from build123d import *
from build123d.topology import SkipClean

# Parameters (mm, degrees)
BOSS_EXTRUDE1_DEPTH  = 2
BOSS_EXTRUDE2_START  = 4.75
BOSS_EXTRUDE2_DEPTH  = 4.75
BOSS_EXTRUDE3_START  = 2
SKETCH3_R            = 1.7
BOSS_EXTRUDE3_DEPTH  = 2
SKETCH4_R            = 2.2
SKETCH4_R_2          = 1.7
BOSS_EXTRUDE4_DEPTH  = 0.5
CHAMFER1_SIZE        = 0.5
SKETCH5_W            = 7.5
SKETCH5_H            = 3
BOSS_EXTRUDE5_DEPTH  = 2
BOSS_EXTRUDE6_DEPTH  = 6.75
BOSS_EXTRUDE8_DEPTH  = 6.75
SKETCH10_W           = 15
SKETCH10_H           = 3
BOSS_EXTRUDE9_DEPTH  = 15
SKETCH11_R           = 1.65
CUT_EXTRUDE1_DEPTH   = 22.34244597
FILLET1_START        = -3
FILLET1_DEPTH        = 7.75
CHAMFER6_SIZE        = 1.5
BOSS_EXTRUDE11_START = -6.75
BOSS_EXTRUDE11_DEPTH = 6.75
BOSS_EXTRUDE12_REACH = 29.029
SKETCH16_W           = 15
SKETCH16_H           = 1.5
CUT_EXTRUDE3_DEPTH   = 0.5
SKETCH17_W           = 15
SKETCH17_H           = 1.5
CUT_EXTRUDE4_DEPTH   = 15
CHAMFER8_SIZE        = 1


with BuildPart() as part:
    # Sketch1 → Boss-Extrude1 (new body)
    with BuildSketch(Plane.XY):
        with BuildLine():
            Line((4.594082841, 4.876925553), (5.159993549, 5.442836262))
            ThreePointArc((5.159993549, 5.442836262), (0, 7.5), (-5.159993549, 5.442836262))
            Line((-5.159993549, 5.442836262), (-4.594082841, 4.876925553))
            ThreePointArc((-4.594082841, 4.876925553), (0, 6.7), (4.594082841, 4.876925553))
        make_face()
    extrude(amount=-BOSS_EXTRUDE1_DEPTH)

    # Sketch1<3> → Boss-Extrude2 (add)
    with BuildSketch(Plane.XY.offset(BOSS_EXTRUDE2_START)):
        with BuildLine():
            Line((4.594082841, 4.876925553), (5.159993549, 5.442836262))
            ThreePointArc((5.159993549, 5.442836262), (0, 7.5), (-5.159993549, 5.442836262))
            Line((-5.159993549, 5.442836262), (-4.594082841, 4.876925553))
            ThreePointArc((-4.594082841, 4.876925553), (0, 6.7), (4.594082841, 4.876925553))
        make_face()
        with BuildLine():
            Line((4.454772721, 4.454772721), (4.596194078, 4.596194078))
            Line((4.596194078, 4.596194078), (5.303300859, 5.303300859))
            ThreePointArc((5.303300859, 5.303300859), (5.232112384, 5.373546315), (5.159993549, 5.442836262))
            Line((5.159993549, 5.442836262), (4.594082841, 4.876925553))
            ThreePointArc((4.594082841, 4.876925553), (0, 6.7), (-4.594082841, 4.876925553))
            Line((-4.594082841, 4.876925553), (-5.159993549, 5.442836262))
            ThreePointArc((-5.159993549, 5.442836262), (-5.232112384, 5.373546315), (-5.303300859, 5.303300859))
            Line((-5.303300859, 5.303300859), (-4.596194078, 4.596194078))
            Line((-4.596194078, 4.596194078), (-4.454772721, 4.454772721))
            ThreePointArc((-4.454772721, 4.454772721), (0, 6.3), (4.454772721, 4.454772721))
        make_face()
    extrude(amount=-BOSS_EXTRUDE2_DEPTH)

    # Sketch3 → Boss-Extrude3 (add)
    with BuildSketch(Plane.XY.offset(4.75).offset(BOSS_EXTRUDE3_START)):
        with BuildLine():
            ThreePointArc((5.303300859, 5.303300859), (0, 7.5), (-5.303300859, 5.303300859))
            Line((-5.303300859, 5.303300859), (-2.792750347, -1.095694072))
            ThreePointArc((-2.792750347, -1.095694072), (0, -3), (2.792750347, -1.095694072))
            Line((2.792750347, -1.095694072), (5.303300859, 5.303300859))
        make_face()
        Circle(SKETCH3_R, mode=Mode.SUBTRACT)
    extrude(amount=-BOSS_EXTRUDE3_DEPTH)

    # Sketch4 → Boss-Extrude4 (add)
    with SkipClean():  # the faces are left unmerged after this step: merging them gives an invalid solid
        with BuildSketch(Plane(origin=(0, 0, 4.75), x_dir=(-1, 0, 0), z_dir=(0, 0, -1))):
            with Locations(Location((0, 0, 0), (0, 0, 180))):
                Circle(SKETCH4_R)
            Circle(SKETCH4_R_2, mode=Mode.SUBTRACT)
        extrude(amount=BOSS_EXTRUDE4_DEPTH)
    add(part.part.scale(1), mode=Mode.REPLACE)  # the faces are merged on a copy

    # Chamfer1
    chamfer1_edges = [part.edges().sort_by_distance(p)[0] for p in [
        (-2.2, 0, 4.75),
    ]]
    chamfer(chamfer1_edges, length=CHAMFER1_SIZE - 0.0001)  # a hair under: the kernel refuses the full size

    # Sketch5 → Boss-Extrude5 (add)
    with BuildSketch(Plane.XY.offset(6.75)):
        with BuildLine():
            ThreePointArc((-5.303300859, 5.303300859), (-2.870125743, 6.929096494), (0, 7.5))
            Line((0, 7.5), (-7.5, 7.5))
            Line((-7.5, 7.5), (-2.634698995, -1.434698995))
            ThreePointArc((-2.634698995, -1.434698995), (-2.71901318, -1.26766215), (-2.792750347, -1.095694072))
            Line((-2.792750347, -1.095694072), (-5.303300859, 5.303300859))
        make_face()
        with Locations((-3.75, 9)):
            Rectangle(SKETCH5_W, SKETCH5_H)
        with Locations((3.75, 9)):
            Rectangle(SKETCH5_W, SKETCH5_H)
        with BuildLine():
            Line((7.5, 7.5), (0, 7.5))
            ThreePointArc((0, 7.5), (2.870125743, 6.929096494), (5.303300859, 5.303300859))
            Line((5.303300859, 5.303300859), (2.792750347, -1.095694072))
            ThreePointArc((2.792750347, -1.095694072), (2.740333064, -1.220890945), (2.682306676, -1.343588812))
            Line((2.682306676, -1.343588812), (7.5, 7.5))
        make_face()
    extrude(amount=-BOSS_EXTRUDE5_DEPTH)

    # Sketch6 → Boss-Extrude6 (add)
    with BuildSketch(Plane(origin=(0, 0, 4.75), x_dir=(-1, 0, 0), z_dir=(0, 0, -1))):
        with BuildLine():
            Line((-5.921621025, 4.602651891), (-5.499242594, 3.827313795))
            ThreePointArc((-5.499242594, 3.827313795), (-5.138626065, 4.299362995), (-4.737615434, 4.737615434))
            Line((-4.737615434, 4.737615434), (-5.303300859, 5.303300859))
            ThreePointArc((-5.303300859, 5.303300859), (-5.623383774, 4.962615735), (-5.921621025, 4.602651891))
        make_face()
        with BuildLine():
            ThreePointArc((4.737615434, 4.737615434), (5.13888851, 4.2990493), (5.499709828, 3.826642367))
            Line((5.499709828, 3.826642367), (5.922007367, 4.602154794))
            ThreePointArc((5.922007367, 4.602154794), (5.623592059, 4.962379707), (5.303300859, 5.303300859))
            Line((5.303300859, 5.303300859), (4.737615434, 4.737615434))
        make_face()
    extrude(amount=BOSS_EXTRUDE6_DEPTH)

    # Sketch8 → Boss-Extrude8 (add)
    with BuildSketch(Plane(origin=(0, 0, 4.75), x_dir=(-1, 0, 0), z_dir=(0, 0, -1))):
        with BuildLine():
            Line((5.922007367, 4.602154794), (7.5, 7.5))
            Line((7.5, 7.5), (7.5, 10.5))
            Line((7.5, 10.5), (-7.5, 10.5))
            Line((-7.5, 10.5), (-7.5, 7.5))
            Line((-7.5, 7.5), (-5.921621025, 4.602651891))
            ThreePointArc((-5.921621025, 4.602651891), (0.000314788, 7.499999993), (5.922007367, 4.602154794))
        make_face()
    extrude(amount=BOSS_EXTRUDE8_DEPTH)

    # Sketch10 → Boss-Extrude9 (add)
    with BuildSketch(Plane(origin=(0, 0, -2), x_dir=(-1, 0, 0), z_dir=(0, 0, -1))):
        with Locations((0, 9)):
            Rectangle(SKETCH10_W, SKETCH10_H)
    extrude(amount=BOSS_EXTRUDE9_DEPTH)

    # Sketch11 → Cut-Extrude1 (cut, through all)
    with BuildSketch(Plane.XZ.offset(-7.5)):
        with Locations(Location((0, -9.5, 0), (0, 0, 270))):
            Circle(SKETCH11_R)
    extrude(amount=-CUT_EXTRUDE1_DEPTH, mode=Mode.SUBTRACT)

    # Fillet1: read off the stored shape, not the designer's step
    # Fillet1 outline → Fillet1 (cut)
    with BuildSketch(Plane.XY.offset(FILLET1_START)):
        with BuildLine():
            ThreePointArc((-5.316260804, 4.077667356), (-5.490505676, 3.999994233), (-5.650601756, 4.10374217))
            Line((-5.650601756, 4.10374217), (-5.499709828, 3.826642367))
            ThreePointArc((-5.499709828, 3.826642367), (-5.409441613, 3.953219123), (-5.316260804, 4.077667356))
        make_face()
        with BuildLine():
            ThreePointArc((5.650134675, 4.104298532), (5.49004858, 4.000580786), (5.315823507, 4.078237419))
            ThreePointArc((5.315823507, 4.078237419), (5.408988293, 3.953839354), (5.499242594, 3.827313795))
            Line((5.499242594, 3.827313795), (5.650134675, 4.104298532))
        make_face()
    extrude(amount=FILLET1_DEPTH, mode=Mode.SUBTRACT)

    # Chamfer6
    chamfer6_edges = [part.edges().sort_by_distance(p)[0] for p in [
        (7.5, 10.5, -5.125),
        (-7.5, 10.5, -5.125),
    ]]
    chamfer(chamfer6_edges, length=CHAMFER6_SIZE)

    # Sketch12 → Boss-Extrude11 (add)
    with BuildSketch(Plane(origin=(0, 0, -2), x_dir=(-1, 0, 0), z_dir=(0, 0, -1)).offset(BOSS_EXTRUDE11_START)):
        with BuildLine():
            Line((-5.303300859, 5.303300859), (-5.210007514, 5.210007514))
            ThreePointArc((-5.210007514, 5.210007514), (-5.138810365, 5.280244751), (-5.066666421, 5.349509134))
            Line((-5.066666421, 5.349509134), (-5.159993549, 5.442836262))
            ThreePointArc((-5.159993549, 5.442836262), (-5.232112384, 5.373546315), (-5.303300859, 5.303300859))
        make_face()
        with BuildLine():
            ThreePointArc((-5.315823507, 4.078237419), (-5.49004858, 4.000580786), (-5.650134675, 4.104298532))
            Line((-5.650134675, 4.104298532), (-5.283538928, 3.431357806))
            ThreePointArc((-5.283538928, 3.431357806), (0.000460722, 6.299999983), (5.284040746, 3.430584993))
            Line((5.284040746, 3.430584993), (5.650601756, 4.10374217))
            ThreePointArc((5.650601756, 4.10374217), (5.490505675, 3.999994233), (5.316260804, 4.077667356))
            ThreePointArc((5.316260804, 4.077667356), (5.037756417, 4.417126926), (4.737615434, 4.737615434))
            Line((4.737615434, 4.737615434), (5.210007514, 5.210007514))
            ThreePointArc((5.210007514, 5.210007514), (5.138810365, 5.280244751), (5.066666421, 5.349509134))
            Line((5.066666421, 5.349509134), (4.594082841, 4.876925553))
            ThreePointArc((4.594082841, 4.876925553), (0, 6.7), (-4.594082841, 4.876925553))
            Line((-4.594082841, 4.876925553), (-5.066666421, 5.349509134))
            ThreePointArc((-5.066666421, 5.349509134), (-5.138810365, 5.280244751), (-5.210007514, 5.210007514))
            Line((-5.210007514, 5.210007514), (-4.737615434, 4.737615434))
            ThreePointArc((-4.737615434, 4.737615434), (-5.037519576, 4.41739703), (-5.315823507, 4.078237419))
        make_face()
        with BuildLine():
            Line((-5.85264511, 4.476036395), (-5.650134675, 4.104298532))
            ThreePointArc((-5.650134675, 4.104298532), (-5.49004858, 4.000580786), (-5.315823507, 4.078237419))
            ThreePointArc((-5.315823507, 4.078237419), (-5.037519576, 4.41739703), (-4.737615434, 4.737615434))
            Line((-4.737615434, 4.737615434), (-5.210007514, 5.210007514))
            ThreePointArc((-5.210007514, 5.210007514), (-5.543487095, 4.85366948), (-5.85264511, 4.476036395))
        make_face()
        with BuildLine():
            Line((5.159993549, 5.442836262), (5.066666421, 5.349509134))
            ThreePointArc((5.066666421, 5.349509134), (5.138810365, 5.280244751), (5.210007514, 5.210007514))
            Line((5.210007514, 5.210007514), (5.303300859, 5.303300859))
            ThreePointArc((5.303300859, 5.303300859), (5.232112384, 5.373546315), (5.159993549, 5.442836262))
        make_face()
        with BuildLine():
            ThreePointArc((5.316260804, 4.077667356), (5.490505675, 3.999994233), (5.650601756, 4.10374217))
            Line((5.650601756, 4.10374217), (5.853045643, 4.47551263))
            ThreePointArc((5.853045643, 4.47551263), (5.543704265, 4.853421435), (5.210007514, 5.210007514))
            Line((5.210007514, 5.210007514), (4.737615434, 4.737615434))
            ThreePointArc((4.737615434, 4.737615434), (5.037756417, 4.417126926), (5.316260804, 4.077667356))
        make_face()
    extrude(amount=BOSS_EXTRUDE11_DEPTH)

    # Boss-Extrude12: up to this face of the body (flat: up to its plane)
    boss_extrude12_end = Plane(part.part.faces().sort_by_distance((-0.00029363, 5.45528482, 6.75))[0])
    # Sketch16 → Boss-Extrude12 (add, up to the picked face)
    with BuildSketch(Plane(origin=(0, 0, -17), x_dir=(-1, 0, 0), z_dir=(0, 0, -1)), mode=Mode.PRIVATE) as boss_extrude12_sk1:
        with Locations((0, 9.75)):
            Rectangle(SKETCH16_W, SKETCH16_H)
    boss_extrude12_tool1 = split(extrude(boss_extrude12_sk1.sketch, amount=-BOSS_EXTRUDE12_REACH, mode=Mode.PRIVATE), bisect_by=boss_extrude12_end, keep=Keep.BOTH, mode=Mode.PRIVATE)
    add(boss_extrude12_tool1.solids().sort_by(Axis((0, 9.75, -17), (0, 0, 1)))[0])

    # Sketch13 → Cut-Extrude3 (cut)
    with BuildSketch(Plane.XY.offset(6.75)):
        with BuildLine():
            ThreePointArc((3.4124071, 2.086978147), (-0.000677338, 3.999999943), (-3.413113698, 2.085822351))
            Line((-3.413113698, 2.085822351), (-6.5, 7.754618569))
            Line((-6.5, 7.754618569), (-6.5, 8.585786438))
            Line((-6.5, 8.585786438), (-5.585786438, 9.5))
            Line((-5.585786438, 9.5), (5.585786438, 9.5))
            Line((5.585786438, 9.5), (6.5, 8.585786438))
            Line((6.5, 8.585786438), (6.5, 7.754711685))
            Line((6.5, 7.754711685), (3.4124071, 2.086978147))
        make_face()
    extrude(amount=-CUT_EXTRUDE3_DEPTH, mode=Mode.SUBTRACT)

    # Sketch17 → Cut-Extrude4 (cut)
    with BuildSketch(Plane(origin=(0, 0, -17), x_dir=(-1, 0, 0), z_dir=(0, 0, -1))):
        with Locations((0, 9.75)):
            Rectangle(SKETCH17_W, SKETCH17_H)
    extrude(amount=-CUT_EXTRUDE4_DEPTH, mode=Mode.SUBTRACT)

    # Chamfer8
    chamfer8_edges = [part.edges().sort_by_distance(p)[0] for p in [
        (7.5, 10.5, 2.375),
        (-7.5, 10.5, 2.375),
    ]]
    chamfer(chamfer8_edges, length=CHAMFER8_SIZE)


solid = part.part
Check sheet for the modelled part. Datum: model origin and axes. Units: mm. A direction names the side the tool comes from. Give positions to 0.01 mm unless a question says otherwise; leave off trailing zeros. Write each loop counter-clockwise with the first axis right and the second up, starting at its lowest first coordinate (ties: lowest second). Pieces come first, ordered by that corner, then holes. Notation, with made-up numbers: (56, 38) -> (82, 38) arc R24 cw to (82, 56) -> close; hole circle Ø7 at (65.5, 52.25). An arc over 180 degrees is marked (long way). One line per item, written item: value. Start each with the question number.
Item 1: Section check C-C on z = 2.75. Record the cut outline in (x, y).
Item 2: Tool access check on faces 4 (the flat face through (0.1, 7.5, -7.7)), 5 (the flat face through (0.1, 9, -11.3)), 6 (the flat face through (0, 7, 6.25)), 7 (the flat face through (7.5, 8, -5)). Record the directions out of +Z, -Z, +X, -X, +Y, -Y that give a thin tool (end or side, any length) a straight path to the whole face; none if there is none.
Item 3: Gauge pin test, flat ends, axial feed: pin 1 (3 mm diameter, centred on x = -0.5, y = 2.5, fed in from -Z); pin 2 (0.8 mm diameter, centred on x = 0, y = 10, fed in from -Z); pin 3 (1.5 mm diameter, centred on x = -1, z = -3, fed in from +Y). Record the tip position at first contact, or that the pin passes through.
Item 4: Draft check along X on faces 1 (the flat face through (7, 10, 2)), 2 (the flat face through (0, 10, -2)), 3 (the flat face through (0, 3, 4.75)). Enter one of: +X half, -X half, draft (parallel to the pull), parting line (faces both ways), or undercut.
Item 5: Material ranges on probe 1 along Y at (x, z) = (0, 4.55); probe 2 along X at (y, z) = (8.55, -9.5); probe 3 along Y at (x, z) = (0, 5.4), recorded low to high. Write a range as from..to.
Item 6: Section check B-B on x = 0. State how many separate pieces and enclosed holes the cut face has, then the cut area to 3 significant figures.
Item 7: Section check A-A on z = -9.5. Record the cut outline in (x, y).
Results list:
1. outline: (-7.5, 7.5) -> (-5.28, 3.43) arc R6.3 cw to (5.28, 3.43) -> (7.5, 7.5) -> (7.5, 9.5) -> (6.5, 10.5) -> (-6.5, 10.5) -> (-7.5, 9.5) -> close
2. face 4: -Z, +X, -X, -Y
2. face 5: -Z, +X, -X, +Y
2. face 6: +Z
2. face 7: +Z, -Z, +X, +Y, -Y
3. pin 1: z = 4.25
3. pin 2: z = -2
3. pin 3: y = 9
4. face 1: +X half
4. face 2: draft
4. face 3: undercut
5. probe 1: -2.5..-1.7, 1.7..2.5, 6.3..10.5
5. probe 2: -7.5..-1.65, 1.65..7.5
5. probe 3: -3..-1.7, 1.7..10.5
6. separate pieces: 3
6. enclosed holes: 0
6. area: 64.1 mm²
7. outline: (-7.5, 7.5) -> (-1.65, 7.5) -> (-1.65, 9) -> (-7.5, 9) -> close; (1.65, 7.5) -> (7.5, 7.5) -> (7.5, 9) -> (1.65, 9) -> close
